```python
from build123d import *

# Parameters (mm, degrees)
SKETCH1_R           = 3
BOSS_EXTRUDE1_DEPTH = 2


with BuildPart() as part:
    # Sketch1 → Boss-Extrude1 (new body)
    with BuildSketch(Plane(origin=(0, 0, 0), x_dir=(1, 0, 0), z_dir=(0, 1, 0))):
        with BuildLine():
            Line((25.842346039, -10.014425763), (6.693666426, -0.919624764))
            ThreePointArc((6.693666426, -0.919624764), (5.113423812, 0.145118135), (4.046267677, 1.723732067))
            ThreePointArc((4.046267677, 1.723732067), (-4.027578724, 1.766958961), (1.471755352, -4.144571212))
            ThreePointArc((1.471755352, -4.144571212), (3.304406882, -3.858859691), (5.115110957, -4.26084658))
            Line((5.115110957, -4.26084658), (25.845891994, -14.02203976))
            ThreePointArc((25.845891994, -14.02203976), (27.271804068, -14.304213396), (28.662988426, -13.882961353))
            Line((28.662988426, -13.882961353), (56.254370384, 2.608150475))
            Line((56.254370384, 2.608150475), (56.254370384, 6.608150475))
            Line((56.254370384, 6.608150475), (28.668534032, -9.879646796))
            ThreePointArc((28.668534032, -9.879646796), (27.272327122, -10.30114258), (25.842346039, -10.014425763))
        make_face()
        Circle(SKETCH1_R, mode=Mode.SUBTRACT)
    extrude(amount=BOSS_EXTRUDE1_DEPTH)


solid = part.part
```
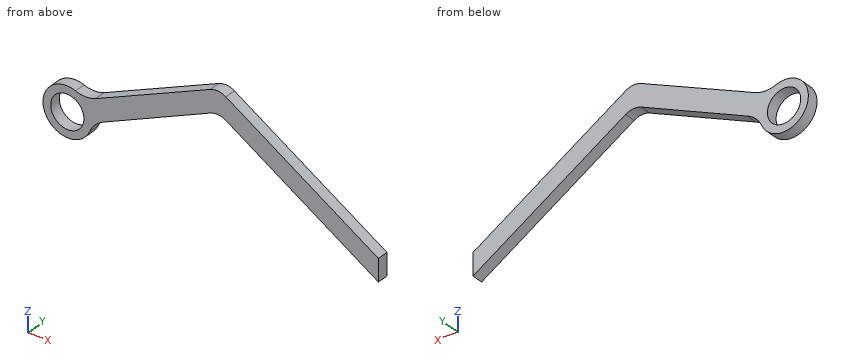
The model under review builds one solid part; all positions refer to its coordinate system, in mm. Give positions to 0.01 mm unless a question says otherwise; leave off trailing zeros. Order: outer loops, then holes, each group sorted by start corner. A loop starts at its lowest first (then second) coordinate and runs counter-clockwise, first axis right, second up. Notation, with made-up numbers: (38, -33.5) - (97, -33.5) arc R15 cw to (97, -12.5) - close; hole circle Ø9 at (-33.75, 32.5). An arc over 180 degrees is marked (long way). Use CSV: the item, a comma, the result in double quotes. Start each with the question number.
Q1. We need section A-A, the plane x = 0. Write out the cut boundary in (y, z), and give its area (3 significant figures).
Q2. We need section C-C, the plane y = 1.4. Write out the cut boundary in (x, z).
Q3. Clearance check with flat-ended pins moving along their axes: pin 1 Ø5 at (x, z) = (0, 0) entering from -Y; pin 2 Ø1 at (x, y) = (4, 1) entering from -Z. State where each tip first meets the part, or that it passes through.
Q4. We need section B-B, the plane z = 0. Write out the cut boundary in (x, y) (3 decimals), and give its area (3 significant figures).
Q5. To check wall thickness, follow line 1 along Z through (x, y) = (0, 1.3); line 2 along X through (y, z) = (0.7, 0) (3 decimals); line 3 along X through (y, z) = (0.7, 2). State the ranges of each line that lie inside material, in increasing order. Write a range as [from, to].
Q6. We need section D-D, the plane z = 6.75. Write out the cut boundary in (x, y), and give its area (3 significant figures).
Outcome:
1,outline,"(0, -4.4) - (2, -4.4) - (2, -3) - (0, -3) - close; (0, 3) - (2, 3) - (2, 4.4) - (0, 4.4) - close"
1,area,"5.59 mm^2"
2,outline,"(1.47, 4.14) arc R4.4 ccw (long way) to (4.05, -1.72) arc R5 cw to (6.69, 0.92) - (25.84, 10.01) arc R3 cw to (28.67, 9.88) - (56.25, -6.61) - (56.25, -2.61) - (28.66, 13.88) arc R3 ccw to (25.85, 14.02) - (5.12, 4.26) arc R5 cw to start; hole circle Ø6 at (0, 0)"
3,pin 1,"passes through"
3,pin 2,"stops at z = -2.66"
4,outline,"(-4.398, 0) - (-3, 0) - (-3, 2) - (-4.398, 2) - close; (3, 0) - (5.265, 0) - (5.265, 2) - (3, 2) - close; (45.198, 0) - (51.891, 0) - (51.891, 2) - (45.198, 2) - close"
4,area,"20.7 mm^2"
5,line 1,"z = [-4.4, -3], [3, 4.4]"
5,line 2,"x = [-4.398, -3], [3, 5.265], [45.198, 51.891]"
5,line 3,"x = [-3.92, -2.24], [2.24, 8.97], [41.85, 48.54]"
6,outline,"(10.4, 0) - (18.97, 0) - (18.97, 2) - (10.4, 2) - close; (33.9, 0) - (40.6, 0) - (40.6, 2) - (33.9, 2) - close"
6,area,"30.5 mm^2"
